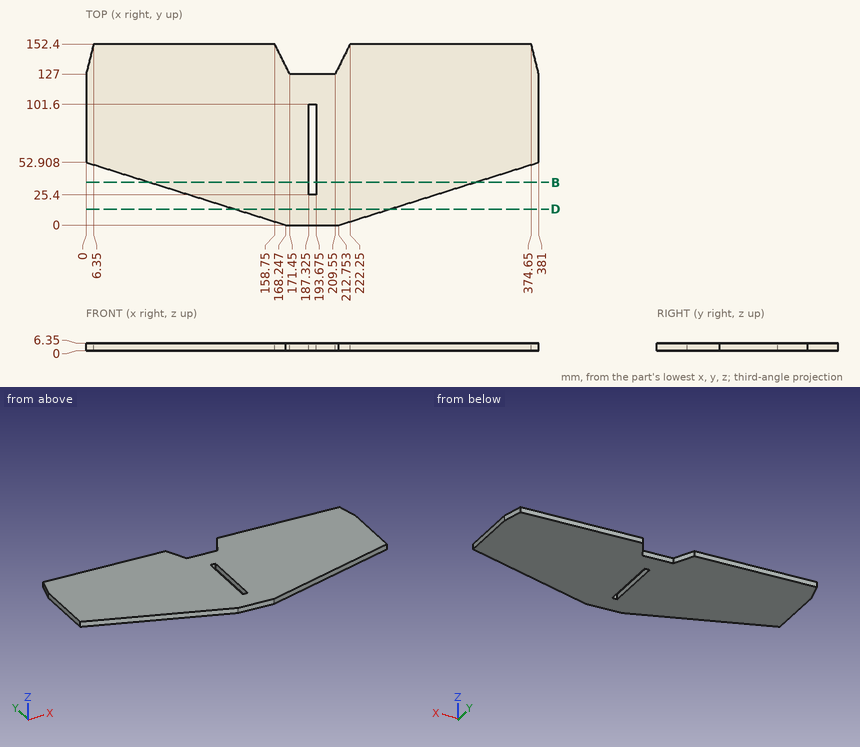
Geometry check sheet. Reference: drawing and pictorial views, mm from the part's lowest x, y, z. Round coordinates to 2 decimals unless told otherwise and drop trailing zeros. Order: outer loops, then holes, each group sorted by start corner. A loop starts at its lowest first (then second) coordinate and runs counter-clockwise, first axis right, second up. Notation, with made-up numbers: M 79.25,-7 L 100.25,-7 A22 ccw 100.25,7 Z; hole C 50,21.5 d1. An arc over 180 degrees is marked long. Answer in a Markdown table with one row per item.
(1) Sectioned sample at D-D, the plane y = 13.5. Record the cut outline in (x, z).
Responses:
| item | result |
|---|---|
| outline | M 125.32,0 L 255.68,0 L 255.68,6.35 L 125.32,6.35 Z |
(2) Go/stop test with flat-tipped pins: P1, Ø1.5, axis at x = 273, z = 5.5, coming from the -Y side; P2, Ø3, axis at x = 191.5, z = 4, coming from the +Y side. Record where each tip stops, or that it passes through.
Responses:
| item | result |
|---|---|
| P1 | stops at y = 18.71 |
| P2 | stops at y = 127 |
(3) Scan lines: probe 1 along Y at (x, z) = (189, 4.25); probe 2 along X at (y, z) = (63.5, 3.5) (3 decimals); probe 3 along Y at (x, z) = (200, 5). Record each from-to range of solid material in increasing order. Write a range as from..to.
Responses:
| item | result |
|---|---|
| probe 1 | y = 0..25.4, 101.6..127 |
| probe 2 | x = 0..187.325, 193.675..381 |
| probe 3 | y = 0..127 |
(4) Sectioned sample at B-B, the plane y = 36. Record the cut outline in (x, z) (3 decimals).
Responses:
| item | result |
|---|---|
| outline | M 53.767,0 L 187.325,0 L 187.325,6.35 L 53.767,6.35 Z; M 193.675,0 L 327.233,0 L 327.233,6.35 L 193.675,6.35 Z |
